```python
from build123d import *

# Parameters (mm, degrees)
F0_W     = 101.6
F0_H     = 101.6
F1_DEPTH = 25.4
F2_W     = 9.6067792356
F2_H     = 19.6575643495
F2_W_2   = 23.4931828454
F2_H_2   = 10.5259682656
F2_W_3   = 8.0198350638
F2_H_3   = 12.465775013
F2_H_4   = 41.7123902589
F2_W_4   = 11.6157357857
F2_H_5   = 18.2192062081
F3_DEPTH = 25.4


# Not quite as in the source:
# - ends of sketch curves that miss each other by under 0.0002 mm in the source are joined


with BuildPart() as f1:
    # F0 (on Top) → F1 (new body)
    with BuildSketch(Plane.XY):
        with Locations((2.876713872, 11.2423545628)):
            Rectangle(F0_W, F0_H)
    extrude(amount=F1_DEPTH)

    # F2 (on face) → F3 (join)
    with BuildSketch(Plane.XY.offset(25.4)):
        Polygon((-31.8836160004, 25.1464881003), (-31.8836160004, 62.0423545628), (-47.923286128, 62.0423545628), (-47.923286128, 25.1464881003), (-39.9034510642, 25.1464881003), align=None)
        Polygon((0, 32.8177288175), (0, 40.0095209479), (0, 48.1602139771), (-13.1849600002, 48.1602139771), (-13.1849600002, 32.8177288175), align=None)
        Polygon((15.5822057277, 40.0095209479), (30.4452423006, 40.0095209479), (30.4452423006, 48.1602139771), (0, 48.1602139771), (0, 40.0095209479), align=None)
        Polygon((42.0609780863, 29.4615607709), (53.676713872, 29.4615607709), (53.676713872, 40.0095209479), (30.4452423006, 40.0095209479), (15.5822057277, 40.0095209479), (15.5822057277, 29.4615607709), align=None)
        Polygon((30.4452423006, -4.1001341306), (30.4452423006, 11.2423545628), (9.8287723958, 11.2423505634), (9.8287723958, -4.1001341306), align=None)
        Polygon((44.0699346364, -9.3741128221), (53.676713872, -9.3741128221), (53.676713872, 11.2423545628), (42.0609780863, 11.2423545628), (30.4452423006, 11.2423545628), (30.4452423006, -4.1001341306), (30.4452423006, -9.3741128221), (42.0609780863, -9.3741128221), align=None)
        with Locations((48.8733242542, -19.2028949969)):
            Rectangle(F2_W, F2_H)
        Polygon((53.676713872, -39.5576454372), (53.676713872, -29.0316771716), (44.0699346364, -29.0316771716), (42.0609780863, -29.0316771716), (-8.390433155, -29.0316771716), (-8.390433155, -39.5576454372), align=None)
        with Locations((-20.1370245777, -34.2946613044)):
            Rectangle(F2_W_2, F2_H_2)
        with Locations((-43.9133685961, -22.7987896651)):
            Rectangle(F2_W_3, F2_H_3)
        Polygon((-47.923286128, -39.5576454372), (-31.8836160004, -39.5576454372), (-31.8836160004, -29.0316771716), (-39.9034510642, -29.0316771716), (-47.923286128, -29.0316771716), align=None)
        with Locations((-43.9133685961, 4.2902929708)):
            Rectangle(F2_W_3, F2_H_4)
        with Locations((47.8688459791, 20.3519576668)):
            Rectangle(F2_W_4, F2_H_5)
    extrude(amount=F3_DEPTH)


solid = f1.part
```
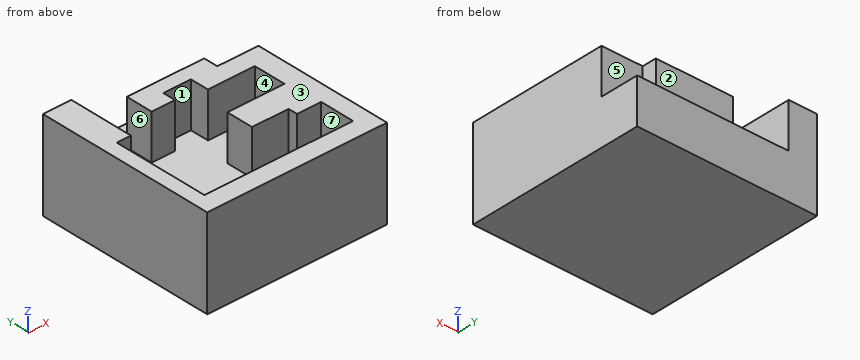
Could you check a few things on this model? Use its own coordinates, in mm. Face numbers are marked on the shaded views. A direction names the side the tool comes from. Round coordinates to 2 decimals unless told otherwise and drop trailing zeros. Write each loop counter-clockwise with the first axis right and the second up, starting at its lowest first coordinate (ties: lowest second). Pieces come first, ordered by that corner, then holes. Notation, with made-up numbers: M 55,78 L 112,78 A19 ccw 112,108 Z; hole C 24.5,-26.75 d1. An arc over 180 degrees is marked long. Answer in a Markdown table with one row per item. Add a question column.
Q1. Imagine slicing it at A-A (x = -6.5). Please give me the cut outline in (y, z).
Q2. Will these pins go through, and if not, where does the flat tip stop? pin 1 Ø1.5 at (x, z) = (-21, 37) entering from +Y; pin 2 Ø1 at (x, y) = (-32.5, 34) entering from -Z; pin 3 Ø4 at (x, z) = (35.5, 35) entering from +Y; pin 4 Ø12 at (y, z) = (51, 32) entering from +X.
Q3. If we mould it in two halves opening along Y, with no side actions, what happens to the marked faces 1, 2, 3 and 4? For each: +Y half, -Y half, draft (parallel to the pull), parting line (faces both ways), or undercut.
Q4. Imagine slicing it at D-D (x = 36). Please give me the cut outline in (y, z), then the cut area to 3 significant figures.
Q5. Imagine slicing it at C-C (z = 36). Please give me the cut outline in (x, y).
Q6. On a 3-axis mill with a long thin cutter (end or side, diameter ignored), from which of +Z, -Z, +X, -X, +Y, -Y can I reach the whole of each face in a straight line? I mean the marked faces 5, 6 and 7. Say none if no direction works.
Q7. If I drill on line 1 (Y direction, x = 13, z = 38.5); line 2 (Y direction, x = 18, z = 45); line 3 (Y direction, x = -37.5, z = 37), over which ranges is the centre line in solid material (lowest first)? Write a range as from..to.
Q8. Imagine slicing it at B-B (y = -11). Please give me the cut outline in (x, z).
Values:
| question | item | result |
|---|---|---|
| 1 | outline | M -39.56,0 L 62.04,0 L 62.04,25.4 L 48.16,25.4 L 48.16,50.8 L 32.82,50.8 L 32.82,25.4 L -29.03,25.4 L -29.03,50.8 L -39.56,50.8 Z |
| 2 | pin 1 | y = -29.03 |
| 2 | pin 2 | z = 0 |
| 2 | pin 3 | y = 40.01 |
| 2 | pin 4 | x = 30.45 |
| 3 | face 1 | undercut |
| 3 | face 2 | +Y half |
| 3 | face 3 | draft |
| 3 | face 4 | undercut |
| 4 | outline | M -39.56,0 L 62.04,0 L 62.04,25.4 L 40.01,25.4 L 40.01,50.8 L 29.46,50.8 L 29.46,25.4 L 11.24,25.4 L 11.24,50.8 L -9.37,50.8 L -9.37,25.4 L -29.03,25.4 L -29.03,50.8 L -39.56,50.8 Z |
| 4 | area | 3,640 mm^2 |
| 5 | outline | M -47.92,-39.56 L 53.68,-39.56 L 53.68,40.01 L 30.45,40.01 L 30.45,48.16 L -13.18,48.16 L -13.18,32.82 L 0,32.82 L 0,40.01 L 15.58,40.01 L 15.58,29.46 L 42.06,29.46 L 42.06,11.24 L 30.45,11.24 L 9.83,11.24 L 9.83,-4.1 L 30.45,-4.1 L 30.45,-9.37 L 44.07,-9.37 L 44.07,-29.03 L -39.9,-29.03 L -39.9,25.15 L -31.88,25.15 L -31.88,62.04 L -47.92,62.04 Z |
| 6 | face 5 | +Z, +X, +Y |
| 6 | face 6 | +Z, +Y |
| 6 | face 7 | +Z |
| 7 | line 1 | -39.56..-29.03, -4.1..11.24, 40.01..48.16 |
| 7 | line 2 | -39.56..-29.03, -4.1..11.24, 29.46..48.16 |
| 7 | line 3 | -39.56..-29.03, 25.15..62.04 |
| 8 | outline | M -47.92,0 L 53.68,0 L 53.68,50.8 L 44.07,50.8 L 44.07,25.4 L -39.9,25.4 L -39.9,50.8 L -47.92,50.8 Z |
